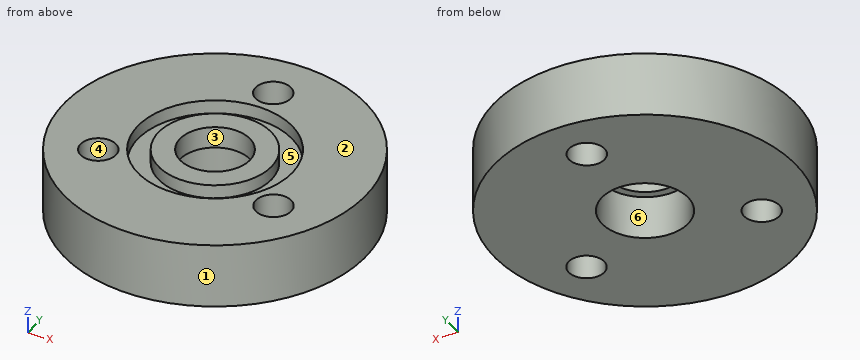
from build123d import *

# Parameters (mm, degrees)
F0_R     = 14
F0_R_2   = 1.65
F0_R_3   = 4
F0_R_4   = 3.25
F1_DEPTH = 6
F2_W     = 1.92
F2_H     = 1.27
F4_DEPTH = 4


with BuildPart() as f1:
    # F0 (on Top) → F1 (new body)
    with BuildSketch(Plane.XY):
        Circle(F0_R)
        with Locations((-8.227241, -4.75)):
            Circle(F0_R_2, mode=Mode.SUBTRACT)
        with Locations((8.227241, -4.75)):
            Circle(F0_R_2, mode=Mode.SUBTRACT)
        Circle(F0_R_3, mode=Mode.SUBTRACT)
        with Locations((0, 9.5)):
            Circle(F0_R_2, mode=Mode.SUBTRACT)
        Circle(F0_R_3)
        Circle(F0_R_4, mode=Mode.SUBTRACT)
    extrude(amount=F1_DEPTH)

    # F2 (on Right) → F3 (revolve, cut)
    with BuildSketch(Plane.YZ):
        with Locations((6.2, 5.365)):
            Rectangle(F2_W, F2_H)
    revolve(axis=Axis((0, 0, 1.894894), (0, 0, -1)), mode=Mode.SUBTRACT)

    # F0 (on Top) → F4 (cut)
    with BuildSketch(Plane.XY):
        Circle(F0_R_3)
        Circle(F0_R_4, mode=Mode.SUBTRACT)
    extrude(amount=F4_DEPTH, mode=Mode.SUBTRACT)


solid = f1.part
Source: CAD feature listing. Evaluate the final solid. Frame: model axes, mm. Face numbers are marked on the shaded views. A direction names the side the tool comes from. Coordinates: 2 decimals unless noted, no trailing zeros. Loops run counter-clockwise (first coordinate to the right, second up) from the corner with the lowest first, then second, coordinate; pieces in that order, holes last. Notation, with made-up numbers: (57, 69.25) -> (114, 69.25) arc R11 cw to (114, 87.25) -> close; hole circle Ø4 at (69.5, 58). An arc over 180 degrees is marked (long way). Answer in a Markdown table with one row per item. Add a question column.
Q1. Contact query for a flat-ended pin moving along its axis: pin 1 Ø2 at (y, z) = (-4, 5) entering from +X. Output: stop coordinate, or through.
Q2. Reachability of the marked faces 4, 5 and 6 from +Z, -Z, +X, -X, +Y, -Y: full face, straight path, thin tool, end or side. Return the list, or none.
Q3. Pull-direction query (Y, two-part tool) for the marked faces 1, 2 and 3; classes: pulls with the +Y half, pulls with the -Y half, needs draft (parallel to the pull), parting line crosses it, or undercut.
Q4. Ray query, line 1 along Y through (x, z) = (0, 2.15); line 2 along Y through (x, z) = (0, 4.6); line 3 along Y through (x, z) = (1.75, 5.65). Return the intervals inside material, ascending.
Q5. Section B-B on y = 0. Return the cut outline in (x, z), and give its area (3 significant figures).
Q6. Section D-D on z = 3.1. Return the cut outline in (x, y).
Q7. Section A-A on z = 5.3. Return the cut outline in (x, y), and give its area (3 significant figures).
Q8. Section C-C on x = 0. Return the cut outline in (y, z).
Computed values:
| question | item | result |
|---|---|---|
| 1 | pin 1 | stops at x = 13.67 |
| 2 | face 4 | +Z, -Z |
| 2 | face 5 | +Z |
| 2 | face 6 | -Z |
| 3 | face 1 | parting line crosses it |
| 3 | face 2 | needs draft |
| 3 | face 3 | undercut |
| 4 | line 1 | y = -14 to -4, 4 to 7.85, 11.15 to 14 |
| 4 | line 2 | y = -14 to -3.25, 3.25 to 7.85, 11.15 to 14 |
| 4 | line 3 | y = -13.89 to -6.94, -4.94 to -2.74, 2.74 to 4.94, 6.94 to 13.89 |
| 5 | outline | (-14, 0) -> (-4, 0) -> (-4, 4) -> (-3.25, 4) -> (-3.25, 6) -> (-5.24, 6) -> (-5.24, 4.73) -> (-7.16, 4.73) -> (-7.16, 6) -> (-14, 6) -> close; (3.25, 4) -> (4, 4) -> (4, 0) -> (14, 0) -> (14, 6) -> (7.16, 6) -> (7.16, 4.73) -> (5.24, 4.73) -> (5.24, 6) -> (3.25, 6) -> close |
| 5 | area | 118 mm^2 |
| 6 | outline | circle Ø28 at (0, 0); hole circle Ø3.3 at (-8.23, -4.75); hole circle Ø8 at (0, 0); hole circle Ø3.3 at (0, 9.5); hole circle Ø3.3 at (8.23, -4.75) |
| 7 | outline | circle Ø28 at (0, 0); circle Ø10.48 at (0, 0); hole circle Ø3.3 at (-8.23, -4.75); hole circle Ø14.32 at (0, 0); hole circle Ø6.5 at (0, 0); hole circle Ø3.3 at (0, 9.5); hole circle Ø3.3 at (8.23, -4.75) |
| 7 | area | 482 mm^2 |
| 8 | outline | (-14, 0) -> (-4, 0) -> (-4, 4) -> (-3.25, 4) -> (-3.25, 6) -> (-5.24, 6) -> (-5.24, 4.73) -> (-7.16, 4.73) -> (-7.16, 6) -> (-14, 6) -> close; (3.25, 4) -> (4, 4) -> (4, 0) -> (7.85, 0) -> (7.85, 6) -> (7.16, 6) -> (7.16, 4.73) -> (5.24, 4.73) -> (5.24, 6) -> (3.25, 6) -> close; (11.15, 0) -> (14, 0) -> (14, 6) -> (11.15, 6) -> close |
